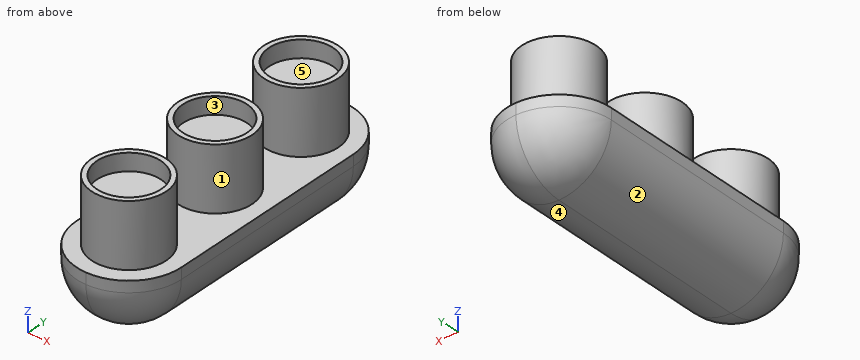
```python
from build123d import *

# Parameters (mm, degrees)
SKETCH1_W           = 16.5
SKETCH1_H           = 49.5
BOSS_EXTRUDE1_DEPTH = 20
SKETCH2_R           = 5.85
SKETCH2_R_2         = 5.05
CUT_EXTRUDE1_DEPTH  = 10
FILLET1_R           = 8.25
SKETCH5_R           = 5.1
BOSS_EXTRUDE2_DEPTH = 7.3


with BuildPart() as part:
    # Sketch1 → Boss-Extrude1 (new body)
    with BuildSketch(Plane.XY):
        with Locations((-57.75, 140.25)):
            Rectangle(SKETCH1_W, SKETCH1_H)
    extrude(amount=BOSS_EXTRUDE1_DEPTH)

    # Sketch2 → Cut-Extrude1 (cut)
    # profile 1 of 8: a face of its own
    with BuildSketch(Plane.XY.offset(20)):
        with BuildLine():
            ThreePointArc((-63.6, 140.25), (-57.75, 146.1), (-51.9, 140.25))
            Line((-51.9, 140.25), (-49.5, 140.25))
            Line((-49.5, 140.25), (-49.5, 165))
            Line((-49.5, 165), (-66, 165))
            Line((-66, 165), (-66, 140.25))
            Line((-66, 140.25), (-63.6, 140.25))
        make_face()
        with Locations((-57.75, 156.75)):
            Circle(SKETCH2_R, mode=Mode.SUBTRACT)
    # profile 2 of 8: a face of its own
    with BuildSketch(Plane.XY.offset(20)):
        with BuildLine():
            Line((-49.5, 140.25), (-51.9, 140.25))
            ThreePointArc((-51.9, 140.25), (-57.75, 134.4), (-63.6, 140.25))
            Line((-63.6, 140.25), (-66, 140.25))
            Line((-66, 140.25), (-66, 115.5))
            Line((-66, 115.5), (-49.5, 115.5))
            Line((-49.5, 115.5), (-49.5, 140.25))
        make_face()
        with Locations((-57.75, 123.75)):
            Circle(SKETCH2_R, mode=Mode.SUBTRACT)
    # profile 3 of 8: a face of its own
    with BuildSketch(Plane.XY.offset(20)):
        with Locations((-57.75, 156.75)):
            Circle(SKETCH2_R_2)
    # profile 4 of 8: a face of its own
    with BuildSketch(Plane.XY.offset(20)):
        with BuildLine():
            ThreePointArc((-62.8, 140.25), (-57.75, 135.2), (-52.7, 140.25))
            Line((-52.7, 140.25), (-62.8, 140.25))
        make_face()
    # profile 5 of 8: a face of its own
    with BuildSketch(Plane.XY.offset(20)):
        with BuildLine():
            Line((-62.8, 140.25), (-52.7, 140.25))
            ThreePointArc((-52.7, 140.25), (-57.75, 145.3), (-62.8, 140.25))
        make_face()
    # profile 6 of 8: a face of its own
    with BuildSketch(Plane.XY.offset(20)):
        with BuildLine():
            ThreePointArc((-62.8, 140.25), (-57.75, 135.2), (-52.7, 140.25))
            Line((-52.7, 140.25), (-62.8, 140.25))
        make_face()
    # profile 7 of 8: a face of its own
    with BuildSketch(Plane.XY.offset(20)):
        with BuildLine():
            Line((-62.8, 140.25), (-52.7, 140.25))
            ThreePointArc((-52.7, 140.25), (-57.75, 145.3), (-62.8, 140.25))
        make_face()
    # profile 8 of 8: a face of its own
    with BuildSketch(Plane.XY.offset(20)):
        with Locations((-57.75, 123.75)):
            Circle(SKETCH2_R_2)
    extrude(amount=-CUT_EXTRUDE1_DEPTH, mode=Mode.SUBTRACT)

    # Fillet1
    fillet1_edges = [part.edges().sort_by_distance(p)[0] for p in [
        (-57.75, 165, 0),
    ]]
    fillet(fillet1_edges, radius=FILLET1_R)
    fillet1_2_edges = [part.edges().sort_by_distance(p)[0] for p in [
        (-49.5, 136.125, 0),
    ]]
    fillet(fillet1_2_edges, radius=FILLET1_R)
    fillet1_3_edges = [part.edges().sort_by_distance(p)[0] for p in [
        (-61.875, 115.5, 0),
    ]]
    fillet(fillet1_3_edges, radius=FILLET1_R)
    fillet1_4_edges = [part.edges().sort_by_distance(p)[0] for p in [
        (-66, 140.25, 0),
    ]]
    fillet(fillet1_4_edges, radius=FILLET1_R - 0.0001)  # a hair under: the kernel refuses the full size

    # Sketch5 → Boss-Extrude2 (add)
    with BuildSketch(Plane.XY.offset(10)):
        with Locations((-57.75, 156.75)):
            Circle(SKETCH5_R)
        with Locations((-57.75, 140.25)):
            Circle(SKETCH5_R)
        with Locations((-57.75, 123.75)):
            Circle(SKETCH5_R)
    extrude(amount=BOSS_EXTRUDE2_DEPTH)


solid = part.part
```
The listing builds one solid part. Answer for the finished solid, in the listing's coordinates (mm). Face numbers are marked on the shaded views. A direction names the side the tool comes from. Round coordinates to 2 decimals unless told otherwise and drop trailing zeros. Return JSON: item names as keys, results as strings. Group by question number.
1. Which of the six approach directions +Z, -Z, +X, -X, +Y, -Y give full straight-line access (tool end or side, diameter ignored) to the marked faces 4 and 5?
2. Each of these flat-tipped pins is pushed along its axis until it touches: P1, Ø3, axis at x = -59, y = 139.5, coming from the +Z side; P2, Ø5, axis at y = 138.5, z = 4, coming from the +X side; P3, Ø1.5, axis at y = 125, z = 3, coming from the +X side. Where does it stop, or does it pass through?
3. The mould has two halves that part along X. Classify the marked faces 1, 2 and 3: pulls with the +X half, pulls with the -X half, needs draft (parallel to the pull), parting line crosses it, or undercut.
4. Consider probe 1 along Y at (x, z) = (-57.75, 19.45); probe 2 along Y at (x, z) = (-56.25, 16); probe 3 along X at (y, z) = (122, 16). Determine where each line is inside the solid, lowest interval first.
Resolved:
{
 "1": {"face 4": "-Z, +X, +Y, -Y", "face 5": "+Z"},
 "2": {"P1": "stops at z = 17.3", "P2": "stops at x = -49.69", "P3": "stops at x = -50.84"},
 "3": {"face 1": "parting line crosses it", "face 2": "pulls with the -X half", "face 3": "undercut"},
 "4": {"probe 1": "y = 117.9 to 118.7, 128.8 to 129.6, 134.4 to 135.2, 145.3 to 146.1, 150.9 to 151.7, 161.8 to 162.6", "probe 2": "y = 118.1 to 129.4, 134.6 to 145.9, 151.1 to 162.4", "probe 3": "x = -63.33 to -52.17"}
}
